Autodesk Inventor part; units mm, degrees
ref_plane "YZ Plane" through (0, 0, 0) normal (1, 0, 0) x (0, 1, 0)
ref_plane "XZ Plane" through (0, 0, 0) normal (0, 1, 0) x (-1, 0, 0)
ref_plane "XY Plane" through (0, 0, 0) normal (0, 0, 1) x (1, 0, 0)
sketch "Эскиз1" plane through (0, 0, 0) normal (0, 1, 0) x (-1, 0, 0)
  line L0 (0, 0) -> (10, 0)
  line L1 (10, 0) -> (10, -4)
  line L2 (10, -4) -> (30, -4)
  line L3 (30, -4) -> (30, 0)
  line L4 (30, 0) -> (49, 0)
  line L5 (49, 0) -> (49, 9.8)
  line L6 (49, 9.8) -> (53, 9.8)
  line L7 (53, 9.8) -> (53, 19.8)
  line L8 (53, 19.8) -> (40, 19.8)
  line L9 (40, 19.8) -> (40, 15.8)
  line L10 (40, 15.8) -> (15, 15.8)
  line L11 (15, 15.8) -> (15, 19.8)
  line L12 (15, 19.8) -> (0, 19.8)
  line L13 (0, 19.8) -> (0, 0)
  line L14 (0, 0) -> (-10, 0)
  line L15 (-10, 0) -> (-10, -4)
  line L16 (-10, -4) -> (-30, -4)
  line L17 (-30, -4) -> (-30, 0)
  line L18 (-30, 0) -> (-49, 0)
  line L19 (-49, 0) -> (-49, 9.8)
  line L20 (-49, 9.8) -> (-53, 9.8)
  line L21 (-53, 9.8) -> (-53, 19.8)
  line L22 (-53, 19.8) -> (-40, 19.8)
  line L23 (-40, 19.8) -> (-40, 15.8)
  line L24 (-40, 15.8) -> (-15, 15.8)
  line L25 (-15, 15.8) -> (-15, 19.8)
  line L26 (-15, 19.8) -> (0, 19.8)
  dimension "d0" = 20
  dimension "d1" = 4
  dimension "d2" = 20
  dimension "d3" = 19
  dimension "d4" = 19.8
  dimension "d5" = 30
  dimension "d6" = 25
  dimension "d7" = 10
extrude "Выдавливание1" add sketch "Эскиз1" along normal blind 4
sketch "Эскиз3" plane through (49, 0, 9.8) normal (1, 0, 0) x (0, 0, -1)
  line L0 (-10, 4) -> (0, 4)
  line L1 (-10, 4) -> (9.8, 22)
  line L2 (9.8, 4) -> (13.8, 4)
  line L3 (9.8, 22) -> (9.8, 4)
  line L4 (0, 0) -> (9.8, 0)
  line L5 (-10, 4) -> (9.8, 4)
  dimension "d10" = 22
extrude "Выдавливание2" add sketch "Эскиз3" against normal up to surface (98 mm away)
sketch "Эскиз6" plane through (10, 0, 0) normal (0, 0, -1) x (-1, 0, 0)
  line L0 (-39, 22) -> (59, 22)
  line L1 (-25, 22) -> (45, 22)
  line L2 (45, 22) -> (45, 18)
  line L3 (45, 18) -> (-25, 18)
  line L4 (-25, 18) -> (-25, 22)
  line L5 (0, 0) -> (20, 0)
  point P0 (10, 0)
  point P1 (10, 18)
  point P2 (10, 0)
  dimension "d13" = 70
  dimension "d14" = 4
extrude "Выдавливание3" cut sketch "Эскиз6" against normal through all
sketch "Эскиз8" plane through (35, 18, 0) normal (-1, 0, 0) x (0, 0, 1)
  line L0 (0, 4) -> (4.4, 0)
  line L1 (0, 0) -> (0, 4)
  line L2 (0, 0) -> (4.4, 0)
  line L3 (4.4, 0) -> (10, 0)
  line L4 (19.8, -18) -> (19.8, -14)
  line L5 (10, 0) -> (19.8, -14)
  line L6 (19.8, -14) -> (4.4, 0)
  line L7 (19.8, -14) -> (0, 4)
  line L8 (0, -18) -> (0, 4)
  dimension "d17" = 10
extrude "Выдавливание4" add sketch "Эскиз8" along normal up to surface (70 mm away) contours L3 L5 L6
sketch "Эскиз10" plane through (-35, 18, 0) normal (0, 1, 0) x (1, 0, 0)
  line L0 (35, 0) -> (35, -10)
  line L1 (70, -10) -> (0, -10)
  point P0 (60, -5)
  point P1 (35, -5)
  point P2 (10, -5)
  dimension "d27" = 5
  dimension "d28" = 50
hole "Отверстие1" at (25, 18, 5) at (0, 18, 5) at (-25, 18, 5) direction (0, -1, 0) diameter 2.8 depth 8
properties part number "sameSpacer" material "Пластик АБС"
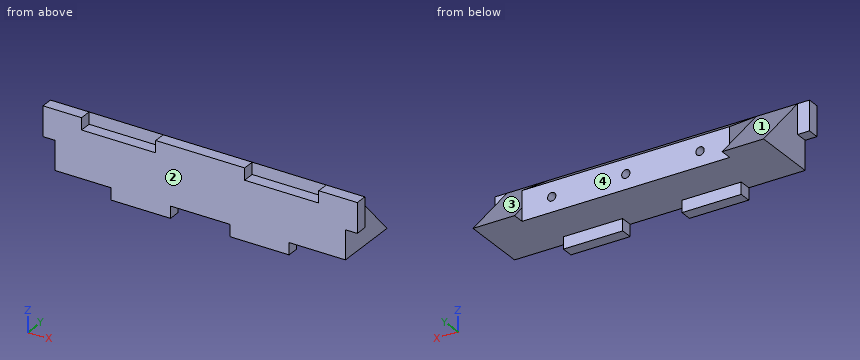
CAD build for the part. Positions are in the model's coordinates, mm. Face numbers are marked on the shaded views. A direction names the side the tool comes from. Round coordinates to 2 decimals unless told otherwise and drop trailing zeros. Write each loop counter-clockwise with the first axis right and the second up, starting at its lowest first coordinate (ties: lowest second). Pieces come first, ordered by that corner, then holes.
(1) Mould opens along X. For the marked faces 3 and 4 say: pulls with the +X half, pulls with the -X half, needs draft (parallel to the pull), parting line crosses it, or undercut.
(2) Probe line 1 along X through (y, z) = (13.25, 5); line 2 along X through (y, z) = (1.25, -0.5); line 3 along Y through (x, z) = (-32, 9). List the from-to ranges inside material, lowest first.
(3) Slice it at D-D, the plane z = 14.25. Write the cut outline in (x, y).
(4) Slice it at B-B, the plane y = 7. Write the cut outline in (x, z).
(5) Slice it at C-C, the plane y = 14.25. Write the cut outline in (x, z) (3 decimals), and give its area (3 significant figures).
(6) Drop flat-ended pins along their axis: P1, Ø2, axis at y = 20.5, z = 2.5, coming from the +X side; P2, Ø12, axis at x = 26, z = 2, coming from the +Y side; P3, Ø1, axis at x = 9.5, y = 18, coming from the -Z side. Give the stop position or say it passes through.
(7) Slice it at A-A, the plane x = 29. Write the cut outline in (y, z).
(8) 3-axis set-ups, long thin cutter, end or side, ignore diameter. For the marked faces 1 and 2: which of +Z, -Z, +X, -X, +Y, -Y reach the whole face in a straight line?
From the geometry:
1. face 3: needs draft
1. face 4: undercut
2. line 1: x = -49 to -26.4, -23.6 to -1.4, 1.4 to 23.6, 26.4 to 49
2. line 2: x = -30 to -10, 10 to 30
2. line 3: y = 0 to 18
3. outline: (-53, 0) - (53, 0) - (53, 4) - (49, 4) - (49, 9.05) - (35, 9.05) - (35, 11.93) - (-35, 11.93) - (-35, 9.05) - (-49, 9.05) - (-49, 4) - (-53, 4) - close
4. outline: (-49, 0) - (49, 0) - (49, 16.5) - (35, 16.5) - (35, 17.7) - (-35, 17.7) - (-35, 16.5) - (-49, 16.5) - close
5. outline: (-49, 0) - (49, 0) - (49, 8.525) - (35, 8.525) - (35, 12.625) - (-35, 12.625) - (-35, 8.525) - (-49, 8.525) - close; hole circle Ø2.8 at (-25, 5); hole circle Ø2.8 at (0, 5); hole circle Ø2.8 at (25, 5)
5. area: 1,100 mm2
6. P1: stops at x = 49
6. P2: stops at y = 18
6. P3: stops at z = 0
7. outline: (0, -4) - (4, -4) - (4, 0) - (18, 0) - (18, 10) - (4, 19.8) - (4, 15.8) - (0, 15.8) - close
8. face 1: +Z, -X, +Y
8. face 2: +Z, -Z, +X, -X, -Y
